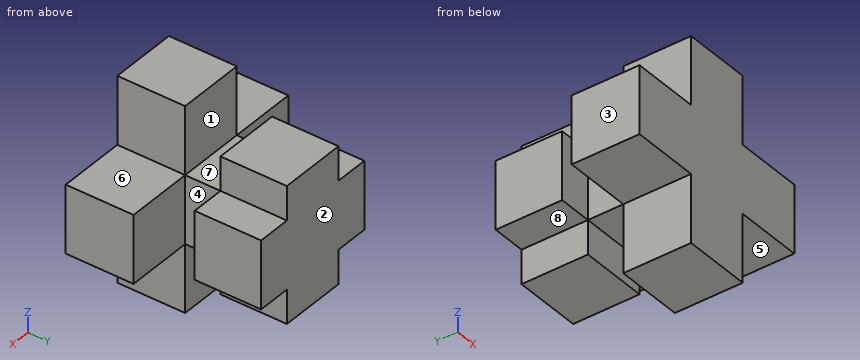
from build123d import *

# Parameters (mm, degrees)
F0_W      = 2
F0_H      = 2
F1_DEPTH  = 5
F2_W      = 2
F2_H      = 2
F3_DEPTH  = 2
F4_W      = 2
F4_H      = 1.958706
F5_DEPTH  = 1
F6_W      = 1.958706
F6_H      = 2
F7_DEPTH  = 1
F8_W      = 2
F8_H      = 2
F9_DEPTH  = 2
F10_W     = 2
F10_H     = 2
F11_DEPTH = 2
F12_W     = 2
F12_H     = 1.958706
F13_DEPTH = 1
F14_W     = 2
F14_H     = 2
F15_DEPTH = 2
F16_W     = 1.958706
F16_H     = 2
F17_DEPTH = 1


with BuildPart() as f1:
    # F0 (on Front) → F1 (new body)
    with BuildSketch(Plane.XZ):
        Rectangle(F0_W, F0_H)
    extrude(amount=F1_DEPTH)

    # F2 (on face) → F3 (join)
    with BuildSketch(Plane(origin=(0, 0, -1), x_dir=(1, 0, 0), z_dir=(0, 0, -1))):
        with Locations((0, 4)):
            Rectangle(F2_W, F2_H)
    extrude(amount=F3_DEPTH)

    # F4 (on face) → F5 (join)
    with BuildSketch(Plane(origin=(0, 0, -1), x_dir=(1, 0, 0), z_dir=(0, 0, -1))):
        with Locations((0, 0.979353)):
            Rectangle(F4_W, F4_H)
    extrude(amount=F5_DEPTH)

    # F6 (on face) → F7 (join)
    with BuildSketch(Plane(origin=(-1, 0, 0), x_dir=(0, -1, 0), z_dir=(-1, 0, 0))):
        with Locations((0.979353, 0)):
            Rectangle(F6_W, F6_H)
    extrude(amount=F7_DEPTH)

    # F8 (on face) → F9 (join)
    with BuildSketch(Plane(origin=(-1, 0, 0), x_dir=(0, -1, 0), z_dir=(-1, 0, 0))):
        with Locations((4, 0)):
            Rectangle(F8_W, F8_H)
    extrude(amount=F9_DEPTH)

    # F10 (on face) → F11 (join)
    with BuildSketch(Plane.XY.offset(1)):
        with Locations((0, -4)):
            Rectangle(F10_W, F10_H)
    extrude(amount=F11_DEPTH)

    # F12 (on face) → F13 (join)
    with BuildSketch(Plane.XY.offset(1)):
        with Locations((0, -0.979353)):
            Rectangle(F12_W, F12_H)
    extrude(amount=F13_DEPTH)

    # F14 (on face) → F15 (join)
    with BuildSketch(Plane.YZ.offset(1)):
        with Locations((-4, 0)):
            Rectangle(F14_W, F14_H)
    extrude(amount=F15_DEPTH)

    # F16 (on face) → F17 (join)
    with BuildSketch(Plane.YZ.offset(1)):
        with Locations((-0.979353, 0)):
            Rectangle(F16_W, F16_H)
    extrude(amount=F17_DEPTH)


solid = f1.part
Design review of the part built by this model. Coordinates are the model's own, in mm. Face numbers are marked on the shaded views. A direction names the side the tool comes from. Round coordinates to 2 decimals unless told otherwise and drop trailing zeros. Order: outer loops, then holes, each group sorted by start corner. A loop starts at its lowest first (then second) coordinate and runs counter-clockwise, first axis right, second up. Notation, with made-up numbers: M -24,59 L 22,59 A33 cw 22,91 Z; hole C -37.5,68 d1. An arc over 180 degrees is marked long. Answer as CSV lines item,"result". Start each with the question number.
1) Add section B-B (y = -1.55). Give the boundary of the cut face in (x, z), then the cut area to 3 significant figures.
2) For pin 1 Ø0.5 at (y, z) = (-2.5, -0.5) entering from -X; pin 2 Ø1.1 at (x, y) = (-1.5, -1) entering from +Z; pin 3 Ø1 at (y, z) = (-3.5, 2) entering from +X, all flat-tipped, find the tip position at first contact; note any pin that passes through.
3) Wall thickness on line 1 along Y through (x, z) = (1.2, 0.85); line 2 along Y through (x, z) = (2.35, 0.65); line 3 along X through (y, z) = (-2.9, -0.1): over which ranges is each line inside the solid? List them lowest first. Write a range as [from, to].
4) Add section C-C (x = 1.25). Give the boundary of the cut face in (y, z), then the cut area to 3 significant figures.
5) Tool access review of the marked faces 4, 5, 6, 7 and 8: name each direction out of +Z, -Z, +X, -X, +Y, -Y from which nothing blocks a thin tool from reaching the whole face with its end or side.
6) The part is to be moulded in two halves that separate along Y. For the marked faces 1, 2 and 3, say which applies: +Y half, -Y half, draft (parallel to the pull), parting line (faces both ways), or undercut.
7) Add section A-A (z = -1.65). Give the boundary of the cut face in (x, y).
8) Add section D-D (x = -0.9). Give the boundary of the cut face in (y, z), then the cut area to 3 significant figures.
Resolved:
1,outline,"M -2,-1 L -1,-1 L -1,-2 L 1,-2 L 1,-1 L 2,-1 L 2,1 L 1,1 L 1,2 L -1,2 L -1,1 L -2,1 Z"
1,area,"12.0 mm^2"
2,pin 1,"x = -1"
2,pin 2,"z = 2"
2,pin 3,"x = 1"
3,line 1,"[-5, -3], [-1.96, 0]"
3,line 2,"[-5, -3]"
3,line 3,"[-1, 1]"
4,outline,"M -5,-1 L -3,-1 L -3,1 L -5,1 Z; M -1.96,-1 L 0,-1 L 0,1 L -1.96,1 Z"
4,area,"7.92 mm^2"
5,face 4,"+Z, -Z, +X"
5,face 5,"-Z, +X, +Y, -Y"
5,face 6,"+Z, +X, +Y, -Y"
5,face 7,"+Z, +X, -X"
5,face 8,"-Z, -X, +Y, -Y"
6,face 1,"undercut"
6,face 2,"+Y half"
6,face 3,"draft"
7,outline,"M -1,-5 L 1,-5 L 1,-3 L -1,-3 Z; M -1,-1.96 L 1,-1.96 L 1,0 L -1,0 Z"
8,outline,"M -5,-3 L -3,-3 L -3,-1 L -1.96,-1 L -1.96,-2 L 0,-2 L 0,2 L -1.96,2 L -1.96,1 L -3,1 L -3,3 L -5,3 Z"
8,area,"21.9 mm^2"
